Work out the finished part from the listing and answer in its coordinate system (mm). A direction names the side the tool comes from. Coordinates: 2 decimals unless noted, no trailing zeros. Write each loop counter-clockwise with the first axis right and the second up, starting at its lowest first coordinate (ties: lowest second). Pieces come first, ordered by that corner, then holes. Notation, with made-up numbers: M 43,52 L 76,52 A33 cw 76,90 Z; hole C -40,29.5 d8. An arc over 180 degrees is marked long. Use CSV: the item, a comma, the result in double quotes.
from build123d import *

# Parameters (mm, degrees)
SKETCH1_W                      = 272
SKETCH1_H                      = 84
BASE_FLANGE1_DEPTH             = 1
EDGE_FLANGE1_STRIP_W           = 5
EDGE_FLANGE1_STRIP_H           = 1
EDGE_FLANGE1_STRIP_CUT_DEPTH   = 272
EDGE_FLANGE1_STRIP_2_W         = 5
EDGE_FLANGE1_STRIP_2_H         = 1
EDGE_FLANGE1_STRIP_CUT_2_DEPTH = 272
EDGE_FLANGE1_DEPTH             = 272
EDGE_FLANGE1_BEND_DEPTH        = 272
CUT_EXTRUDE1_START             = -78.427547771
CUT_EXTRUDE1_DEPTH             = 8.5
CUT_EXTRUDE1_START_2           = 185.072452229
CUT_EXTRUDE1_2_DEPTH           = 8.5
SKETCH13_R                     = 1.6
CUT_EXTRUDE2_DEPTH             = 100
SKETCH14_R                     = 1.5
CUT_EXTRUDE3_DEPTH             = 100


# Read off the part's stored shape, not the designer's step: Cut-Extrude1
# Sheet-metal steps are written as plain solids
with BuildPart() as part:
    # Sketch1 → Base-Flange1 (new body)
    with BuildSketch(Plane(origin=(0, 0, 0), x_dir=(1, 0, 0), z_dir=(0, 1, 0))):
        with Locations((57.572452229, -1.800955414)):
            Rectangle(SKETCH1_W, SKETCH1_H)
    extrude(amount=-BASE_FLANGE1_DEPTH)

    # Edge-Flange1 strip (across the edge) → Edge-Flange1 strip cut (cut)
    with BuildSketch(Plane(origin=(-78.427547771, 0, 43.800955414), x_dir=(0, 0, -1), z_dir=(1, 0, 0))):
        with Locations((-2, -0.5)):
            Rectangle(EDGE_FLANGE1_STRIP_W, EDGE_FLANGE1_STRIP_H)
    extrude(amount=EDGE_FLANGE1_STRIP_CUT_DEPTH, mode=Mode.SUBTRACT)

    # Edge-Flange1 strip 2 (across the edge) → Edge-Flange1 strip cut 2 (cut)
    with BuildSketch(Plane(origin=(193.572452229, 0, -40.199044586), x_dir=(0, 0, 1), z_dir=(-1, 0, 0))):
        with Locations((-2, -0.5)):
            Rectangle(EDGE_FLANGE1_STRIP_2_W, EDGE_FLANGE1_STRIP_2_H)
    extrude(amount=EDGE_FLANGE1_STRIP_CUT_2_DEPTH, mode=Mode.SUBTRACT)

    # Edge-Flange1 section (across the edge) → Edge-Flange1 (add)
    with BuildSketch(Plane(origin=(-78.427547771, 0, 43.800955414), x_dir=(0, 0, -1), z_dir=(1, 0, 0))):
        with BuildLine():
            Line((-1, 0.5), (-1, 23))
            Line((-1, 23), (0, 23))
            Line((0, 23), (0, 0.5))
            ThreePointArc((0, 0.5), (0.146446609, 0.146446609), (0.5, 0))
            Line((0.5, 0), (0.5, -1))
            ThreePointArc((0.5, -1), (-0.560660172, -0.560660172), (-1, 0.5))
        make_face()
    extrude(amount=EDGE_FLANGE1_DEPTH)

    # Edge-Flange1 section 2 (across the edge) → Edge-Flange1 bend (add)
    with BuildSketch(Plane(origin=(193.572452229, 0, -40.199044586), x_dir=(0, 0, 1), z_dir=(-1, 0, 0))):
        with BuildLine():
            Line((-1, 0.5), (-1, 23))
            Line((-1, 23), (0, 23))
            Line((0, 23), (0, 0.5))
            ThreePointArc((0, 0.5), (0.146446609, 0.146446609), (0.5, 0))
            Line((0.5, 0), (0.5, -1))
            ThreePointArc((0.5, -1), (-0.560660172, -0.560660172), (-1, 0.5))
        make_face()
    extrude(amount=EDGE_FLANGE1_BEND_DEPTH)

    # Cut-Extrude1 outline → Cut-Extrude1 (cut)
    with BuildSketch(Plane.YZ.offset(CUT_EXTRUDE1_START)):
        with BuildLine():
            ThreePointArc((0.5, -40.199044586), (0.146446609, -40.052597977), (0, -39.699044586))
            Line((0, -39.699044586), (-1, -39.699044586))
            ThreePointArc((-1, -39.699044586), (-0.560660172, -40.759704758), (0.5, -41.199044586))
            Line((0.5, -41.199044586), (23, -41.199044586))
            Line((23, -41.199044586), (23, -40.199044586))
            Line((23, -40.199044586), (0.5, -40.199044586))
        make_face()
        with BuildLine():
            ThreePointArc((0.5, 44.800955414), (-0.560660172, 44.361615586), (-1, 43.300955414))
            Line((-1, 43.300955414), (0, 43.300955414))
            ThreePointArc((0, 43.300955414), (0.146446609, 43.654508805), (0.5, 43.800955414))
            Line((0.5, 43.800955414), (23, 43.800955414))
            Line((23, 43.800955414), (23, 44.800955414))
            Line((23, 44.800955414), (0.5, 44.800955414))
        make_face()
    extrude(amount=CUT_EXTRUDE1_DEPTH, mode=Mode.SUBTRACT)

    # Cut-Extrude1 2 outline → Cut-Extrude1 2 (cut)
    with BuildSketch(Plane.YZ.offset(CUT_EXTRUDE1_START_2)):
        with BuildLine():
            ThreePointArc((0.5, -40.199044586), (0.146446609, -40.052597977), (0, -39.699044586))
            Line((0, -39.699044586), (-1, -39.699044586))
            ThreePointArc((-1, -39.699044586), (-0.560660172, -40.759704758), (0.5, -41.199044586))
            Line((0.5, -41.199044586), (23, -41.199044586))
            Line((23, -41.199044586), (23, -40.199044586))
            Line((23, -40.199044586), (0.5, -40.199044586))
        make_face()
        with BuildLine():
            ThreePointArc((0.5, 44.800955414), (-0.560660172, 44.361615586), (-1, 43.300955414))
            Line((-1, 43.300955414), (0, 43.300955414))
            ThreePointArc((0, 43.300955414), (0.146446609, 43.654508805), (0.5, 43.800955414))
            Line((0.5, 43.800955414), (23, 43.800955414))
            Line((23, 43.800955414), (23, 44.800955414))
            Line((23, 44.800955414), (0.5, 44.800955414))
        make_face()
    extrude(amount=CUT_EXTRUDE1_2_DEPTH, mode=Mode.SUBTRACT)

    # Sketch13 → Cut-Extrude2 (cut)
    with BuildSketch(Plane(origin=(0, 0, -41.199044586), x_dir=(-1, 0, 0), z_dir=(0, 0, -1))):
        with Locations(Location((-168.072452229, 13, 0), (0, 0, 90))):
            Circle(SKETCH13_R)
        with Locations(Location((-57.572452229, 13, 0), (0, 0, 90))):
            Circle(SKETCH13_R)
        with Locations(Location((52.927547771, 13, 0), (0, 0, 90))):
            Circle(SKETCH13_R)
    extrude(amount=-CUT_EXTRUDE2_DEPTH, mode=Mode.SUBTRACT)

    # Sketch14 → Cut-Extrude3 (cut)
    with BuildSketch(Plane(origin=(0, 0, 0), x_dir=(1, 0, 0), z_dir=(0, 1, 0))):
        with Locations(Location((-74.427547771, -1.800955414, 0), (0, 0, 270))):
            Circle(SKETCH14_R)
        with Locations(Location((-74.427547771, 32.199044586, 0), (0, 0, 270))):
            Circle(SKETCH14_R)
        with Locations(Location((-74.427547771, -35.800955414, 0), (0, 0, 270))):
            Circle(SKETCH14_R)
        with Locations(Location((189.572452229, -35.800955414, 0), (0, 0, 270))):
            Circle(SKETCH14_R)
        with Locations(Location((189.572452229, -1.800955414, 0), (0, 0, 270))):
            Circle(SKETCH14_R)
        with Locations(Location((189.572452229, 32.199044586, 0), (0, 0, 270))):
            Circle(SKETCH14_R)
    extrude(amount=-CUT_EXTRUDE3_DEPTH, mode=Mode.SUBTRACT)


solid = part.part
Item 1: A tool of negligible diameter and unlimited length cuts with its end or side. For faces 4 (the face through (56, -1, 1)), 5 (the face through (59.4, 11.9, -40.199)), from which of +Z, -Z, +X, -X, +Y, -Y can it reach the whole face along a straight path? Write none if from no direction.
Answer:
face 4,"+Z, -Z, +X, -X, -Y"
face 5,"+X, -X, +Y"
Item 2: For a pull along Z with two mould halves and no side action, classify faces 1 (the face through (56, 0, 1)), 2 (the face through (56, 12, 44.801)), 3 (the face through (59.4, 11.6, -41.199)) as released by +Z, released by -Z, zero draft, split by the parting line, or undercut.
Answer:
face 1,"undercut"
face 2,"released by +Z"
face 3,"released by -Z"
Item 3: The part is cut by section A-A (y = 3.5). Write down the section's boundary in (x, z), then the cut area to 3 significant figures.
Answer:
outline,"M -69.93,-41.2 L 185.07,-41.2 L 185.07,-40.2 L -69.93,-40.2 Z; M -69.93,43.8 L 185.07,43.8 L 185.07,44.8 L -69.93,44.8 Z"
area,"510 mm2"
Item 4: The part is cut by section C-C (z = 16). Write down the section's boundary in (x, y).
Answer:
outline,"M -78.43,-1 L 193.57,-1 L 193.57,0 L -78.43,0 Z"
Item 5: The part is cut by section B-B (x = -30.5). Write down the section's boundary in (y, z), then the cut area to 3 significant figures.
Answer:
outline,"M -1,-39.7 A1.5 ccw 0.5,-41.2 L 23,-41.2 L 23,-40.2 L 0.5,-40.2 A0.5 cw 0,-39.7 L 0,43.3 A0.5 cw 0.5,43.8 L 23,43.8 L 23,44.8 L 0.5,44.8 A1.5 ccw -1,43.3 Z"
area,"131 mm2"
Item 6: Given pin 1 (1.9 mm diameter, centred on x = 168.07, y = 13, fed in from -Z); pin 2 (12 mm diameter, centred on x = -22.5, z = 7, fed in from +Y); pin 3 (1.2 mm diameter, centred on y = 6, z = -40.5, fed in from +X); pin 4 (0.8 mm diameter, centred on x = 189, y = -0.5, fed in from -Z), each flat-ended and moving along its own axis, determine where each tip first touches the part or whether it passes through.
Answer:
pin 1,"passes through"
pin 2,"stops at y = 0"
pin 3,"stops at x = 185.07"
pin 4,"stops at z = -39.7"
Item 7: Consider probe 1 along X at (y, z) = (13, -40.9); probe 2 along Z at (x, y) = (148, 4.75); probe 3 along Y at (x, z) = (-48, 17). Determine where each line is inside the solid, lowest interval first.
Answer:
probe 1,"x = -69.93 to -54.53, -51.33 to 55.97, 59.17 to 166.47, 169.67 to 185.07"
probe 2,"z = -41.2 to -40.2, 43.8 to 44.8"
probe 3,"y = -1 to 0"
